Model file for the job. Use its own axes, mm. A direction names the side the tool comes from. Give positions to 0.01 mm unless a question says otherwise; leave off trailing zeros. Loops run counter-clockwise (first coordinate to the right, second up) from the corner with the lowest first, then second, coordinate; pieces in that order, holes last. Notation, with made-up numbers: (23.5, 44) - (67.5, 44) arc R10 cw to (67.5, 49) - close; hole circle Ø11 at (-6, -32). An arc over 180 degrees is marked (long way). Use a Markdown table: item, result.
from build123d import *

# Parameters (mm, degrees)
F1_DEPTH = 40
F2_R     = 4.4
F3_DEPTH = 18
F4_R     = 1
F5_R     = 1
F6_DEPTH = 15


with BuildPart() as f1:
    # F0 (on Right) → F1 (new body)
    with BuildSketch(Plane.YZ):
        with BuildLine():
            Line((0, 0), (0, -18))
            Line((0, -18), (108.1519347629, -18))
            Line((108.1519347629, -18), (110, -18))
            add(Edge.make_bspline(
                [(100, 0), (102.15, -2.75), (110.3054567735, -15.7496706799), (110, -18)],
                knots=[0, 0, 0, 0, 0.5188602886, 0.5188602886, 0.5188602886, 0.5188602886], degree=3))
            Line((100, 0), (0, 0))
        make_face()
    extrude(amount=F1_DEPTH)

    # F2 (on face) → F3 (cut, through all)
    with BuildSketch(Plane.XY):
        with Locations((20, 87.3)):
            Circle(F2_R)
        with Locations((20, 62.4)):
            Circle(F2_R)
        with Locations((20, 37.5)):
            Circle(F2_R)
        with Locations((20, 12.6)):
            Circle(F2_R)
    extrude(amount=-F3_DEPTH, mode=Mode.SUBTRACT)

    # F4
    f4_edges = [f1.edges().sort_by_distance(p)[0] for p in [
        (0, 50, 0),
        (0, 55, -18),
        (40, 50, 0),
        (40, 55, -18),
    ]]
    fillet(f4_edges, radius=F4_R)

    # F5 (on face) → F6 (cut)
    with BuildSketch(Plane(origin=(0, 0, -18), x_dir=(1, 0, 0), z_dir=(0, 0, -1))):
        with Locations((20, -72.9)):
            Circle(F5_R)
        with Locations((20, -29)):
            Circle(F5_R)
    extrude(amount=-F6_DEPTH, mode=Mode.SUBTRACT)


solid = f1.part
(1) Mould opens along Y. For faces 1 (the flat face through (20, 29, -3)), 2 (the cylindrical face through (19.427, 66.763, -8.874)), 3 (the flat face through (20, 51, 0)), 4 (the flat face through (20, 0, -9)) say: pulls with the +Y half, pulls with the -Y half, needs draft (parallel to the pull), parting line crosses it, or undercut.
Computed:
| item | result |
|---|---|
| face 1 | undercut |
| face 2 | undercut |
| face 3 | needs draft |
| face 4 | pulls with the -Y half |
(2) Pin check, flat tip, straight feed: P1, Ø0.6, axis at x = 20, y = 72.5, coming from the -Z side. Stop position of the tip, or through.
Computed:
| item | result |
|---|---|
| P1 | z = -3 |
(3) Drill centre lines: probe 1 along X at (y, z) = (13, -9.5); probe 2 along X at (y, z) = (29, -8.5); probe 3 along Y at (x, z) = (22.5, -1.75). Where is each one in solid material? Low to high. Write a range as [from, to].
Computed:
| item | result |
|---|---|
| probe 1 | [0, 15.62], [24.38, 40] |
| probe 2 | [0, 19], [21, 40] |
| probe 3 | [0, 8.98], [16.22, 33.88], [41.12, 58.78], [66.02, 83.68], [90.92, 101.25] |
(4) Slice it at B-B, the plane x = 20. Count the separate pieces of the cut face and the enclosed holes in it, plus the area to 3 significant figures.
Computed:
| item | result |
|---|---|
| separate pieces | 5 |
| enclosed holes | 0 |
| area | 1,210 mm² |
(5) Slice it at D-D, the plane y = 85.5. Write the cut outline in (x, z).
Computed:
| item | result |
|---|---|
| outline | (0, -17) arc R1 ccw to (1, -18) - (15.99, -18) - (15.99, 0) - (1, 0) arc R1 ccw to (0, -1) - close; (24.01, -18) - (39, -18) arc R1 ccw to (40, -17) - (40, -1) arc R1 ccw to (39, 0) - (24.01, 0) - close |
(6) 3-axis set-ups, long thin cutter, end or side, ignore diameter. For faces 5 (the flat face through (20, 73, -3)), 6 (the cylindrical face through (15.604, 12.793, -8.874)): which of +Z, -Z, +X, -X, +Y, -Y reach the whole face in a straight line?
Computed:
| item | result |
|---|---|
| face 5 | -Z |
| face 6 | +Z, -Z |
(7) Slice it at A-A, the plane y = 37.5. Write the cut outline in (x, z).
Computed:
| item | result |
|---|---|
| outline | (0, -17) arc R1 ccw to (1, -18) - (15.6, -18) - (15.6, 0) - (1, 0) arc R1 ccw to (0, -1) - close; (24.4, -18) - (39, -18) arc R1 ccw to (40, -17) - (40, -1) arc R1 ccw to (39, 0) - (24.4, 0) - close |
